```python
from build123d import *

# Parameters (mm, degrees)
F1_DEPTH = 3.175


with BuildPart() as f1:
    # F0 (on Right) → F1 (new body)
    with BuildSketch(Plane.YZ):
        Polygon((-16.967481, 52.385313), (-29.032481, 52.385313), (-29.032481, 40.320313), (-32.207481, 40.320313), (-32.207481, 24.877113), (-29.032481, 24.877113), (-29.032481, 9.637113), (-32.207481, 9.637113), (-32.207481, -5.806087), (-29.032481, -5.806087), (-29.032481, -17.871087), (-16.967481, -17.871087), (-16.967481, -21.046087), (-1.524281, -21.046087), (-1.524281, -17.871087), (13.715719, -17.871087), (13.715719, -21.046087), (29.158919, -21.046087), (29.158919, -17.871087), (41.223919, -17.871087), (41.223919, -5.806087), (44.398919, -5.806087), (44.398919, 9.637113), (41.223919, 9.637113), (41.223919, 24.877113), (44.398919, 24.877113), (44.398919, 40.320313), (41.223919, 40.320313), (41.223919, 52.385313), (29.158919, 52.385313), (29.158919, 55.560313), (13.715719, 55.560313), (13.715719, 52.385313), (-1.473481, 52.385313), (-1.524281, 55.560313), (-16.967481, 55.560313), align=None)
    extrude(amount=F1_DEPTH)


solid = f1.part
```
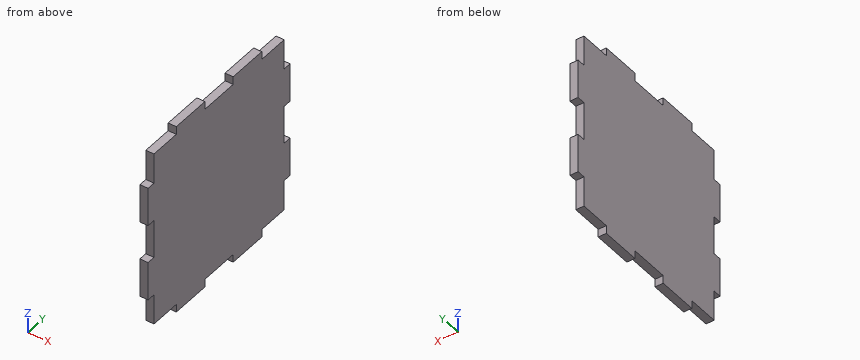
The listing builds one solid part. Answer for the finished solid, in the listing's coordinates (mm). Round coordinates to 2 decimals unless told otherwise and drop trailing zeros. Order: outer loops, then holes, each group sorted by start corner. A loop starts at its lowest first (then second) coordinate and runs counter-clockwise, first axis right, second up. Notation, with made-up numbers: (19, 62) - (75, 62) arc R22 cw to (75, 72) - close; hole circle Ø7 at (-1.5, -6.5). An arc over 180 degrees is marked (long way). Put each result on its own line as item: value. Start each with the question number.
(1) Find section B-B (y = 2). Give the vertices of the cut face in (x, z) (3 decimals).
(2) Given P1, Ø1, axis at x = 1, z = -19, coming from the -Y side; P2, Ø1, axis at x = 2, z = -19.5, coming from the +Y side; P3, Ø1.6, axis at x = 1.5, y = -23.5, coming from the -Z side, each flat-ended and moving along its own axis, determine where each tip first touches the part or whether it passes through.
(3) Straight lines are drawn through the part: probe 1 along Z at (x, y) = (0.65, 3); probe 2 along Y at (x, z) = (2.05, 11.5). For each, find the intervals that lie inside material, in ascending order. Write a range as from..to.
(4) Find section A-A (z = 19.5). Give the vertices of the cut face in (x, y) (3 decimals), plus the area to 3 significant figures.
Reply:
1. outline: (0, -17.871) - (3.175, -17.871) - (3.175, 52.385) - (0, 52.385) - close
2. P1: y = -16.97
2. P2: y = 29.16
2. P3: z = -17.87
3. probe 1: -17.87..52.39
3. probe 2: -29.03..41.22
4. outline: (0, -29.032) - (3.175, -29.032) - (3.175, 41.224) - (0, 41.224) - close
4. area: 223 mm^2
